```python
from build123d import *

# Parameters (mm, degrees)
F1_DEPTH = 63.5
F0_W     = 25.9565819922
F0_H     = 19.05
F2_DEPTH = 25.4
F3_DEPTH = 12.7
F5_R     = 6.35


with BuildPart() as f1:
    # F0 (on Front) → F1 (new body, symmetric)
    with BuildSketch(Plane.XZ):
        Polygon((22.225, 6.35), (-41.275, 6.35), (-41.275, -6.35), (41.275, -6.35), (41.275, 6.35), align=None)
    extrude(amount=F1_DEPTH, both=True)

    # F0 (on Front) → F2 (join, symmetric)
    with BuildSketch(Plane.XZ):
        with BuildLine():
            Line((22.225, 30.3022), (22.225, 6.35))
            Line((22.225, 6.35), (41.275, 6.35))
            Line((41.275, 6.35), (41.275, 30.3022))
            ThreePointArc((41.275, 30.3022), (45.8874824099, 41.4377175901), (57.023, 46.0502))
            Line((57.023, 46.0502), (59.7684180078, 46.0502))
            Line((59.7684180078, 46.0502), (59.7684180078, 65.1002))
            Line((59.7684180078, 65.1002), (57.023, 65.1002))
            ThreePointArc((57.023, 65.1002), (58.0206866195, 65.0858948211), (59.0175529571, 65.042991046))
            add(Edge.make_bspline(
                [(45.498923229, 63.1365792171), (50.2364600679, 64.1417845), (54.78396405, 64.7988002062), (59.0175529571, 65.042991046)],
                knots=[103.0762503935, 103.0762503935, 103.0762503935, 103.0762503935, 116.2044034303, 116.2044034303, 116.2044034303, 116.2044034303], degree=3))
            ThreePointArc((45.498923229, 63.1365792171), (28.6336038504, 50.4253953293), (22.225, 30.3022))
        make_face()
        with Locations((72.7467090039, 55.5752)):
            Rectangle(F0_W, F0_H)
    extrude(amount=F2_DEPTH, both=True)

    # F0 (on Front) → F3 (join, symmetric)
    with BuildSketch(Plane.XZ):
        with BuildLine():
            add(Edge.make_bspline(
                [(-41.275, 6.35), (-40.6099216302, 25.8870106414), (8.301951797, 55.244167303), (45.498923229, 63.1365792171)],
                knots=[0, 0, 0, 0, 103.0762503935, 103.0762503935, 103.0762503935, 103.0762503935], degree=3))
            Line((-41.275, 6.35), (22.225, 6.35))
            Line((22.225, 6.35), (22.225, 30.3022))
            ThreePointArc((22.225, 30.3022), (28.6336038504, 50.4253953293), (45.498923229, 63.1365792171))
        make_face()
    extrude(amount=F3_DEPTH, both=True)

    # F0 (on Front) → F4 (revolve)
    with BuildSketch(Plane.XZ):
        Polygon((85.725, 69.85), (85.725, 65.1002), (85.725, 46.0502), (85.725, 41.275), (110.5684180078, 41.275), (110.5684180078, 69.85), align=None)
    revolve(axis=Axis((85.725, 0, 55.5625), (0, 0, 1)))

    # F5
    f5_edges = [f1.edges().sort_by_distance(p)[0] for p in [
        (-41.275, -63.5, 0),
        (41.275, -63.5, 0),
        (41.275, 63.5, 0),
        (-41.275, 63.5, 0),
    ]]
    fillet(f5_edges, radius=F5_R)


solid = f1.part
```
Could you check a few things on this model? Use its own coordinates, in mm. A direction names the side the tool comes from. Give positions to 0.01 mm unless a question says otherwise; leave off trailing zeros. Order: outer loops, then holes, each group sorted by start corner. A loop starts at its lowest first (then second) coordinate and runs counter-clockwise, first axis right, second up.
Q1. Suppose I cut it at B-B, the plane y = 41.5. Write out the boundary of the cut face in (x, z) (3 decimals), and give its area (3 significant figures).
Q2. We'd pull the mould along X, two halves only. Please class faces 6 (the flat face through (1, -38, 6.35)), 7 (the cylindrical face through (45.766, -0.356, 41.315)), 8 (the cylindrical face through (39.464, -61.59, 0.089)): +X half, -X half, draft (parallel to the pull), parting line (faces both ways), or undercut.
Q3. I'm going to push flat-ended pins straight in: P1, Ø8, axis at x = 17.5, z = 52.5, coming from the -Y side; P2, Ø11, axis at y = 16, z = 10, coming from the +X side (3 decimals); P3, Ø23, axis at x = 76, y = -7.5, coming from the -Z side (3 decimals); P4, Ø5, axis at x = 44.5, z = 34, coming from the -Y side. Where does each tip first touch, or does it pass through?
Q4. If I drill on line 1 along Z through (x, y) = (5, -30); line 2 along Y through (x, z) = (34.5, 46); line 3 along X through (y, z) = (10.5, 2) (3 decimals), over which ranges is the centre line in solid material (lowest first)?
Q5. Suppose I cut it at A-A, the plane x = 64.5. Write out the boundary of the cut face in (y, z) (3 decimals), and give its area (3 significant figures).
Q6. For faces 1 (the flat face through (46, -25.4, 43)), 2 (the flat face through (60.8, -2, 65.1)), 3 (the flat face through (22.225, -19, 18)), 4 (the flat face through (1, 38, 6.35)), 5 (the flat face through (41.275, -1, 8)), which set-ups out of +Z, -Z, +X, -X, +Y, -Y let a thin tool reach every point of the face, with its end or its side?
Q7. Suppose I cut it at C-C, the plane x = 89. Write out the boundary of the cut face in (y, z) (3 decimals), and give its area (3 significant figures).
Solution:
1. outline: (-41.275, -6.35) - (41.275, -6.35) - (41.275, 6.35) - (-41.275, 6.35) - close
1. area: 1,050 mm2
2. face 6: draft
2. face 7: undercut
2. face 8: +X half
3. P1: stops at y = -12.7
3. P2: stops at x = 41.275
3. P3: stops at z = 41.275
3. P4: passes through
4. line 1: z = -6.35 to 6.35
4. line 2: y = -25.4 to 25.4
4. line 3: x = -41.275 to 41.275
5. outline: (-25.4, 46.05) - (-12.911, 46.05) - (-12.911, 41.275) - (12.911, 41.275) - (12.911, 46.05) - (25.4, 46.05) - (25.4, 65.1) - (12.911, 65.1) - (12.911, 69.85) - (-12.911, 69.85) - (-12.911, 65.1) - (-25.4, 65.1) - close
5. area: 1,210 mm2
6. face 1: +Z, +X, -X, -Y
6. face 2: +Z, -X
6. face 3: +Z, -X, -Y
6. face 4: +Z, -X, +Y
6. face 5: -Z, +X, +Y, -Y
7. outline: (-24.627, 41.275) - (24.627, 41.275) - (24.627, 69.85) - (-24.627, 69.85) - close
7. area: 1,410 mm2
